```python
from build123d import *

# Parameters (mm, degrees)
SKETCH1_W           = 71
SKETCH1_H           = 150
BOSS_EXTRUDE1_DEPTH = 5
SKETCH2_W           = 65
SKETCH2_H           = 45
BOSS_EXTRUDE3_DEPTH = 2
LPATTERN1_COUNT     = 3
LPATTERN1_PITCH     = 50
SKETCH3_W           = 69
SKETCH3_H           = 49.5
BOSS_EXTRUDE8_DEPTH = 25
LPATTERN5_COUNT     = 3
LPATTERN5_PITCH     = 50


with BuildPart() as part:
    # Sketch1 → Boss-Extrude1 (new body)
    with BuildSketch(Plane(origin=(0, 0, 0), x_dir=(1, 0, 0), z_dir=(0, 1, 0))):
        Rectangle(SKETCH1_W, SKETCH1_H)
    extrude(amount=BOSS_EXTRUDE1_DEPTH)

    # Sketch2 → Boss-Extrude3 (add)
    with BuildSketch(Plane(origin=(0, 5, 0), x_dir=(1, 0, 0), z_dir=(0, 1, 0))):
        with Locations((0, -50)):
            Rectangle(SKETCH2_W, SKETCH2_H)
    boss_extrude3 = extrude(amount=BOSS_EXTRUDE3_DEPTH)

    # LPattern1: Boss-Extrude3 ×3
    with Locations(*[(0, 0, -i * LPATTERN1_PITCH) for i in range(1, LPATTERN1_COUNT)]):
        add(boss_extrude3)

    # Sketch3 → Boss-Extrude8 (add)
    with BuildSketch(Plane(origin=(0, 7, 0), x_dir=(1, 0, 0), z_dir=(0, 1, 0))):
        with Locations((0, -50.25)):
            Rectangle(SKETCH3_W, SKETCH3_H)
    boss_extrude8 = extrude(amount=BOSS_EXTRUDE8_DEPTH)

    # LPattern5: Boss-Extrude8 ×3
    with Locations(*[(0, 0, -i * LPATTERN5_PITCH) for i in range(1, LPATTERN5_COUNT)]):
        add(boss_extrude8)


solid = part.part
```
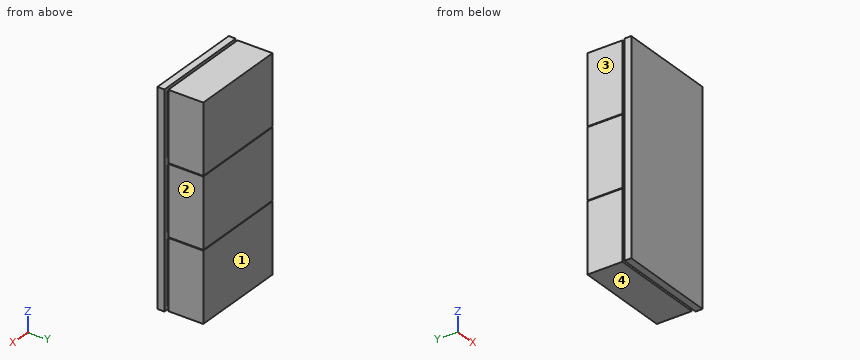
Can you work these out from the model? Positions are in its coordinate system, mm. Face numbers are marked on the shaded views. A direction names the side the tool comes from. Coordinates: 2 decimals unless noted, no trailing zeros. Loops run counter-clockwise (first coordinate to the right, second up) from the corner with the lowest first, then second, coordinate; pieces in that order, holes last.
Item 1: I'm going to push flat-ended pins straight in: pin 1 (12 mm diameter, centred on y = 27.5, z = -34.5, fed in from -X); pin 2 (0.6 mm diameter, centred on x = 13.5, y = 5.5, fed in from +Z); pin 3 (8 mm diameter, centred on y = 21, z = -32.5, fed in from +X); pin 4 (3 mm diameter, centred on x = -8.5, z = -3.5, fed in from -Y). Where does each tip first touch, or does it pass through?
Answers below:
pin 1: stops at x = -34.5
pin 2: stops at z = 72.5
pin 3: stops at x = 34.5
pin 4: stops at y = 0
Item 2: Please list where these lines run through material, in increasing order: L1, parallel to Z at x = -21.5, y = 5.5; L2, parallel to Z at x = -16, y = 19.5; L3, parallel to X at y = 10, z = -11.
Answers below:
L1: z = -72.5 to -27.5, -22.5 to 22.5, 27.5 to 72.5
L2: z = -74.5 to -25, -24.5 to 25, 25.5 to 75
L3: x = -34.5 to 34.5
Item 3: Which directions (+Z, -Z, +X, -X, +Y, -Y) give clear straight access to the entire face, cutting with the end or side of a thin tool? Please do the marked faces 1, 2, 3 and 4.
Answers below:
face 1: +Z, -Z, +X, -X, +Y
face 2: +Z, -Z, +X, +Y
face 3: +Z, -Z, -X, +Y
face 4: -Z, +X, -X, +Y
Item 4: Suppose I cut it at A-A (y = 8.5). Please give me the cut outline in (x, z), then the cut area to 3 significant figures.
Answers below:
outline: (-34.5, -74.5) - (34.5, -74.5) - (34.5, -25) - (-34.5, -25) - close; (-34.5, -24.5) - (34.5, -24.5) - (34.5, 25) - (-34.5, 25) - close; (-34.5, 25.5) - (34.5, 25.5) - (34.5, 75) - (-34.5, 75) - close
area: 10,200 mm2
Item 5: Suppose I cut it at B-B (z = 14). Please give me the cut outline in (x, y), then the cut area to 3 significant figures.
Answers below:
outline: (-35.5, 0) - (35.5, 0) - (35.5, 5) - (32.5, 5) - (32.5, 7) - (34.5, 7) - (34.5, 32) - (-34.5, 32) - (-34.5, 7) - (-32.5, 7) - (-32.5, 5) - (-35.5, 5) - close
area: 2,210 mm2
